Source: CAD feature listing. Evaluate the final solid. Frame: model axes, mm. A direction names the side the tool comes from. Round coordinates to 2 decimals unless told otherwise and drop trailing zeros. Write each loop counter-clockwise with the first axis right and the second up, starting at its lowest first coordinate (ties: lowest second). Pieces come first, ordered by that corner, then holes. Notation, with made-up numbers: M 34.5,-35 L 44.5,-35 A25 ccw 44.5,1 Z; hole C 61.5,22 d8. An arc over 180 degrees is marked long. Answer in a Markdown table with one row per item. Add a question column.
Item 1: Contact query for flat-ended pins moving along their axis: pin 1 (1.5 mm diameter, centred on x = 4, z = 157.5, fed in from +Y); pin 2 (12 mm diameter, centred on y = -42, z = 1.5, fed in from +X); pin 3 (2 mm diameter, centred on x = -26, z = 182, fed in from -Y). Output: stop coordinate, or through.
Item 2: Cut plane D-D on z = 228. Return loops of the section in (x, y), and give its area (3 significant figures).
Item 3: Set-up query: faces 4 (the face through (-16, -17, -32)), 5 (the face through (0, -15, -36)), 6 (the face through (-31.996, -28, 142)). Return all of +Z, -Z, +X, -X, +Y, -Y with unobstructed straight access to the full face (end or side cutting, diameter ignored); none if empty.
Item 4: Mould query, pull axis X, two halves, no side actions, for faces 1 (the face through (0, 8, 145)), 2 (the face through (5.08, 5, 145)), 3 (the face through (-22, 17.888, -38)). Classes: released by +X, released by -X, zero draft, split by the parting line, or undercut.
Item 5: Material intervals for probe 1 along X at (y, z) = (10, 189); probe 2 along Y at (x, z) = (-29, 224); probe 3 along Z at (x, y) = (-14, -27), sorted ascending.
Item 6: Cut plane B-B on z = -12. Return loops of the section in (x, y), and give its area (3 significant figures).
Item 7: Cut plane C-C on x = -21.5. Return loops of the section in (y, z), and give its area (3 significant figures).
Item 8: Cut plane A-A on y = 6. Return loops of the section in (x, z), and give its area (3 significant figures).
from build123d import *

# Parameters (mm, degrees)
BOSS_EXTRUDE1_DEPTH = 288.036
SKETCH2_W           = 5.08
SKETCH2_H           = 5.08
CUT_EXTRUDE1_DEPTH  = 299.722207266
SKETCH3_W           = 12.446
SKETCH3_H           = 70.614516874
SKETCH3_W_2         = 31.996
SKETCH3_H_2         = 5.08
BOSS_EXTRUDE2_DEPTH = 32
SKETCH7_W           = 44.446
SKETCH7_H           = 70.61
BOSS_EXTRUDE3_DEPTH = 12.45


with BuildPart() as part:
    # Sketch1 → Boss-Extrude1 (new body)
    with BuildSketch(Plane.XY):
        Polygon((-44.446, 17.892402527), (-44.446, -52.722114347), (-31.996, -52.722114347), (-31.996, -2.187597473), (5.08, -2.187597473), (5.08, 12.812402527), (0, 12.812402527), (0, 2.892402527), (-32, 2.892402527), (-32, 17.892402527), align=None)
    extrude(amount=BOSS_EXTRUDE1_DEPTH)

    # Sketch2 → Cut-Extrude1 (cut, through all)
    with BuildSketch(Plane(origin=(0, 12.812402527, 0), x_dir=(1, 0, 0), z_dir=(0, 1, 0))):
        with Locations((2.54, -2.54)):
            Rectangle(SKETCH2_W, SKETCH2_H)
    extrude(amount=-CUT_EXTRUDE1_DEPTH, mode=Mode.SUBTRACT)

    # Sketch3 → Boss-Extrude2 (add)
    with BuildSketch(Plane(origin=(0, 0, 0), x_dir=(-1, 0, 0), z_dir=(0, 0, -1))):
        with Locations((38.223, -17.41485591)):
            Rectangle(SKETCH3_W, SKETCH3_H)
        with Locations((15.998, 0.352402527)):
            Rectangle(SKETCH3_W_2, SKETCH3_H_2)
    extrude(amount=BOSS_EXTRUDE2_DEPTH)

    # Sketch7 → Boss-Extrude3 (add)
    with BuildSketch(Plane(origin=(0, 0, -32), x_dir=(-1, 0, 0), z_dir=(0, 0, -1))):
        with Locations((22.223, -17.417114347)):
            Rectangle(SKETCH7_W, SKETCH7_H)
    extrude(amount=BOSS_EXTRUDE3_DEPTH)


solid = part.part
Results below:
| question | item | result |
|---|---|---|
| 1 | pin 1 | y = 12.81 |
| 1 | pin 2 | x = -32 |
| 1 | pin 3 | y = -2.19 |
| 2 | outline | M -44.45,-52.72 L -32,-52.72 L -32,-2.19 L 5.08,-2.19 L 5.08,12.81 L 0,12.81 L 0,2.89 L -32,2.89 L -32,17.89 L -44.45,17.89 Z |
| 2 | area | 1,120 mm2 |
| 3 | face 4 | +Z, +X |
| 3 | face 5 | -Z, +X, +Y, -Y |
| 3 | face 6 | +Z, +X, -Y |
| 4 | face 1 | undercut |
| 4 | face 2 | released by +X |
| 4 | face 3 | zero draft |
| 5 | probe 1 | -44.45 to -32, 0 to 5.08 |
| 5 | probe 2 | -2.19 to 2.89 |
| 5 | probe 3 | -44.45 to -32 |
| 6 | outline | M -44.45,-52.72 L -32,-52.72 L -32,17.89 L -44.45,17.89 Z; M -32,-2.19 L 0,-2.19 L 0,2.89 L -32,2.89 Z |
| 6 | area | 1,040 mm2 |
| 7 | outline | M -52.72,-44.45 L 17.89,-44.45 L 17.89,-32 L 2.89,-32 L 2.89,288.04 L -2.19,288.04 L -2.19,-32 L -52.72,-32 Z |
| 7 | area | 2,500 mm2 |
| 8 | outline | M -44.45,-44.45 L 0,-44.45 L 0,-32 L -32,-32 L -32,288.04 L -44.45,288.04 Z; M 0,5.08 L 5.08,5.08 L 5.08,288.04 L 0,288.04 Z |
| 8 | area | 5,970 mm2 |
